Input: part model. Units: mm. Frame: model coordinates. Face numbers are marked on the shaded views. A direction names the side the tool comes from. Give positions to 0.01 mm unless a question says otherwise; leave off trailing zeros. Loops run counter-clockwise (first coordinate to the right, second up) from the corner with the lowest first, then second, coordinate; pieces in that order, holes last. Notation, with made-up numbers: M 73,-34 L 91,-34 A5 ccw 91,-26 Z; hole C -16,89 d5. An arc over 180 degrees is marked long. Use a Markdown table: item, result. Add a question column.
Autodesk Inventor part; units mm, degrees
ref_plane "YZ Plane" through (0, 0, 0) normal (1, 0, 0) x (0, 1, 0)
ref_plane "XY Plane" through (0, 0, 0) normal (0, 0, 1) x (1, 0, 0)
ref_plane "作業平面2" through (0, 6, 0) normal (0, 1, 0) x (-1, 0, 0)
sketch "スケッチ3" plane through (0, 6, 0) normal (0, 1, 0) x (-1, 0, 0)
  line L0 (4, -4) -> (-4, -4)
  line L1 (-4, -4) -> (-4, 4)
  line L2 (-4, 4) -> (4, 4)
  line L3 (4, 4) -> (4, -4)
  line L4 (4, -4) -> (-4, 4) construction
  line L5 (-4, -4) -> (4, 4) construction
  line L6 (5, -5) -> (-5, -5)
  line L7 (-5, -5) -> (-5, 5)
  line L8 (-5, 5) -> (5, 5)
  line L9 (5, 5) -> (5, -5)
  line L10 (5, -5) -> (-5, 5) construction
  line L11 (-5, -5) -> (5, 5) construction
  point P0 (0, 0)
  point P1 (0, 0)
  dimension "d19" = 8
  dimension "d20" = 8
  dimension "d21" = 10
  dimension "d22" = 10
sketch "スケッチ1" plane through (0, 0, 0) normal (0, 1, 0) x (-1, 0, 0)
  line L0 (6.5, -6.5) -> (-6.5, 6.5) construction
  line L1 (-6.5, -6.5) -> (6.5, 6.5) construction
  line L2 (1.0311, 3.848) -> (3.848, 1.0311)
  line L3 (3.848, 1.0311) -> (2.8169, -2.8169)
  line L4 (2.8169, -2.8169) -> (-1.0311, -3.848)
  line L5 (-1.0311, -3.848) -> (-3.848, -1.0311)
  line L6 (-3.848, -1.0311) -> (-2.8169, 2.8169)
  line L7 (-2.8169, 2.8169) -> (1.0311, 3.848)
  line L8 (-6.5, -6.5) -> (6.5, -6.5)
  line L9 (6.5, -6.5) -> (6.5, 6.5)
  line L10 (6.5, 6.5) -> (-6.5, 6.5)
  line L11 (-6.5, 6.5) -> (-6.5, -6.5)
  line L12 (-6.5, -6.5) -> (6.5, 6.5) construction
  line L13 (6.5, -6.5) -> (-6.5, 6.5) construction
  circle A0 centre (0, 0) radius 2.05
  dimension "d33" = 6.9
  dimension "d34" = 13
  dimension "d35" = 13
  dimension "d36" = 4.1
extrude "押し出し8" add sketch "スケッチ1" along normal blind 6 contours L2 L3 L4 L5 L6 L7 | L11 L10 L9 L8 | A0
extrude "押し出し9" cut sketch "スケッチ3" against normal blind 2
extrude "押し出し10" cut sketch "スケッチ1" along normal blind 3 contours L2 L3 L4 L5 L6 L7
extrude "押し出し11" cut sketch "スケッチ1" along normal blind 6 contours A0
properties part number "pin_joint_ver1"
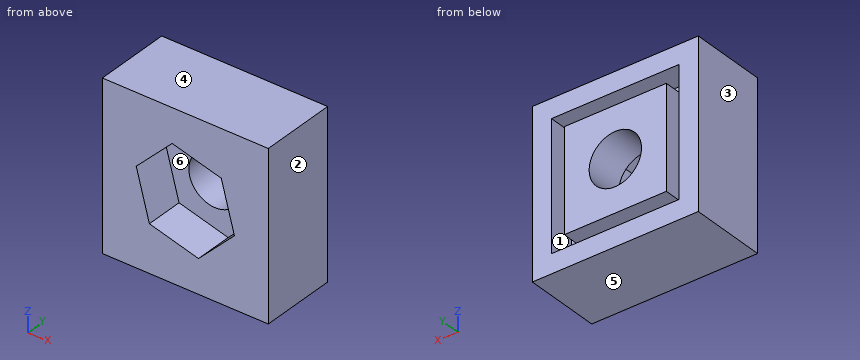
1) Pull-direction query (X, two-part tool) for the marked faces 1, 2, 3 and 4; classes: pulls with the +X half, pulls with the -X half, needs draft (parallel to the pull), parting line crosses it, or undercut.
2) Section query D-D, the plane y = 3.75. Return the cut outline in (x, z).
3) Ray query, line 1 (Z direction, x = 3.75, y = 4.45); line 2 (Z direction, x = 0, y = 4.4). Return the intervals inside material, ascending. Write a range as [from, to].
4) Section query C-C, the plane x = 0. Return the cut outline in (y, z).
5) Reachability of the marked faces 5 and 6 from +Z, -Z, +X, -X, +Y, -Y: full face, straight path, thin tool, end or side. Return the list, or none.
6) Section query A-A, the plane y = 1.05. Return the cut outline in (x, z).
7) Section query B-B, the plane z = 0. Return the cut outline in (x, y), and give its area (3 significant figures).
8) Contact query for flat-ended pins moving along their axis: P1, Ø5, axis at x = 5, z = 4.5, coming from the -Y side; P2, Ø3.5, axis at x = 0, z = 0, coming from the -Y side. Output: stop coordinate, or through.
Entries:
| question | item | result |
|---|---|---|
| 1 | face 1 | undercut |
| 1 | face 2 | pulls with the +X half |
| 1 | face 3 | pulls with the -X half |
| 1 | face 4 | needs draft |
| 2 | outline | M -6.5,-6.5 L 6.5,-6.5 L 6.5,6.5 L -6.5,6.5 Z; hole C 0,0 d4.1 |
| 3 | line 1 | z = [-6.5, -5], [-4, 4], [5, 6.5] |
| 3 | line 2 | z = [-6.5, -5], [-4, -2.05], [2.05, 4], [5, 6.5] |
| 4 | outline | M 0,-6.5 L 6,-6.5 L 6,-5 L 4,-5 L 4,-4 L 6,-4 L 6,-2.05 L 3,-2.05 L 3,-3.57 L 0,-3.57 Z; M 0,3.57 L 3,3.57 L 3,2.05 L 6,2.05 L 6,4 L 4,4 L 4,5 L 6,5 L 6,6.5 L 0,6.5 Z |
| 5 | face 5 | -Z, +X, -X, +Y, -Y |
| 5 | face 6 | -Y |
| 6 | outline | M -6.5,-6.5 L 6.5,-6.5 L 6.5,6.5 L -6.5,6.5 Z; hole M -3.85,1.03 L -2.82,-2.82 L 1.03,-3.85 L 3.85,-1.03 L 2.82,2.82 L -1.03,3.85 Z |
| 7 | outline | M -6.5,0 L -3.57,0 L -3.57,3 L -2.05,3 L -2.05,6 L -4,6 L -4,4 L -5,4 L -5,6 L -6.5,6 Z; M 2.05,3 L 3.57,3 L 3.57,0 L 6.5,0 L 6.5,6 L 5,6 L 5,4 L 4,4 L 4,6 L 2.05,6 Z |
| 7 | area | 40.3 mm² |
| 8 | P1 | stops at y = 0 |
| 8 | P2 | passes through |
